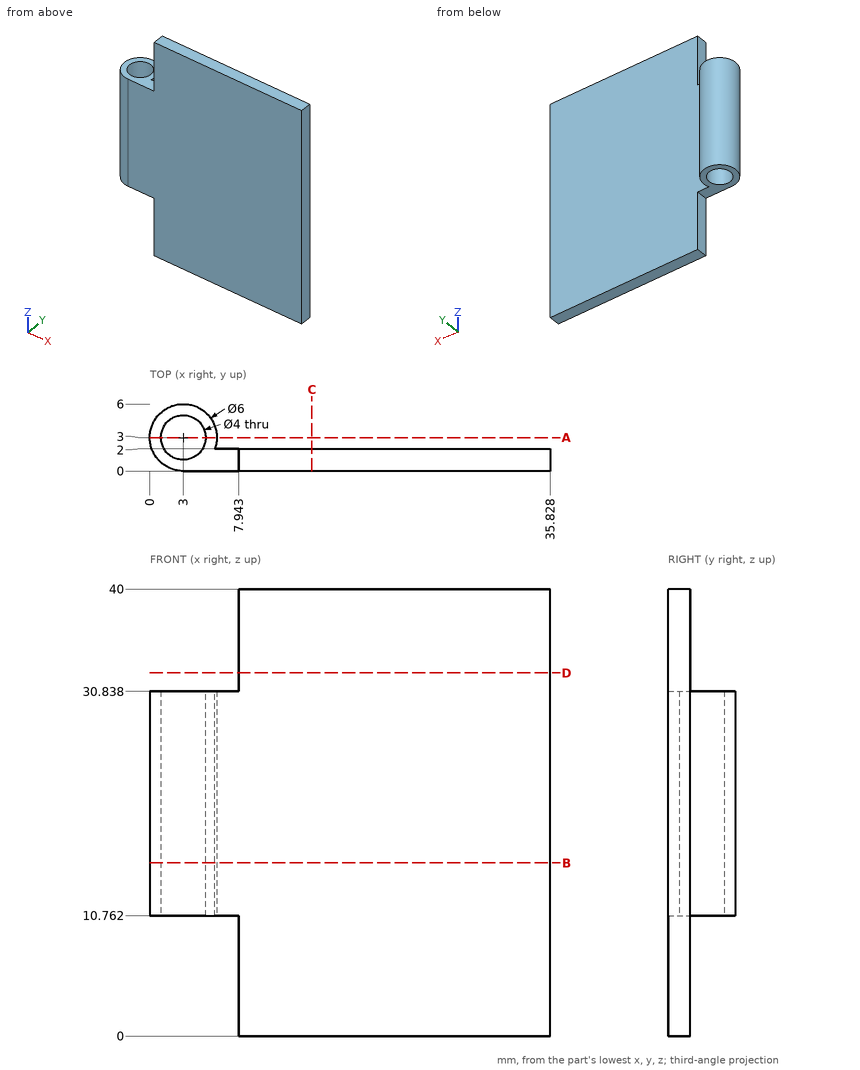
Input: dimensioned drawing with shaded views. Units: mm. Origin: part minimum x, y, z. Give positions to 0.01 mm unless a question says otherwise; leave off trailing zeros. Order: outer loops, then holes, each group sorted by start corner. A loop starts at its lowest first (then second) coordinate and runs counter-clockwise, first axis right, second up. Notation, with made-up numbers: (47, 71) -> (103, 71) arc R35 ccw to (103, 110) -> close; hole circle Ø5 at (-5.5, 16.5). An arc over 180 degrees is marked (long way). Use one line per item in the form item = value.
1) Section D-D, the plane z = 32.5. Return loops of the section in (x, y).
Response values:
outline = (7.94, 0) -> (35.83, 0) -> (35.83, 2) -> (7.94, 2) -> close
2) Section B-B, the plane z = 15.5. Return loops of the section in (x, y).
Response values:
outline = (3, 0) -> (35.83, 0) -> (35.83, 2) -> (5.83, 2) arc R3 ccw (long way) to start; hole circle Ø4 at (3, 3)
3) First-contact query: pin 1 Ø1.8 at (x, y) = (5.5, 4) entering from +Z; pin 2 Ø1 at (y, z) = (1, 36.5) entering from -X; pin 3 Ø3 at (x, y) = (3.5, 2.5) entering from -Z. Flat tips, straight axial feed; report the tip coordinate or a pass-through.
Response values:
pin_1 = 30.84
pin_2 = 7.94
pin_3 = 10.76
4) Section A-A, the plane y = 3. Return loops of the section in (x, z).
Response values:
outline = (0, 10.76) -> (1, 10.76) -> (1, 30.84) -> (0, 30.84) -> close; (5, 10.76) -> (6, 10.76) -> (6, 30.84) -> (5, 30.84) -> close
5) Line query: probe 1 along Y at (x, z) = (19, 37); probe 2 along X at (y, z) = (1.5, 12) (1 decimal); probe 3 along X at (y, z) = (4.25, 24.5) (1 decimal). Output: solid intervals per line, ascending.
Response values:
probe_1 = 0 to 2
probe_2 = 0.4 to 1.7, 4.3 to 35.8
probe_3 = 0.3 to 1.4, 4.6 to 5.7
6) Section C-C, the plane x = 14.5. Return loops of the section in (y, z).
Response values:
outline = (0, 0) -> (2, 0) -> (2, 40) -> (0, 40) -> close
